Can you work these out from the model? Positions are in its coordinate system, mm. Face numbers are marked on the shaded views. Give positions to 0.01 mm unless a question says otherwise; leave off trailing zeros. Answer as a JSON object with one key per item and string values.
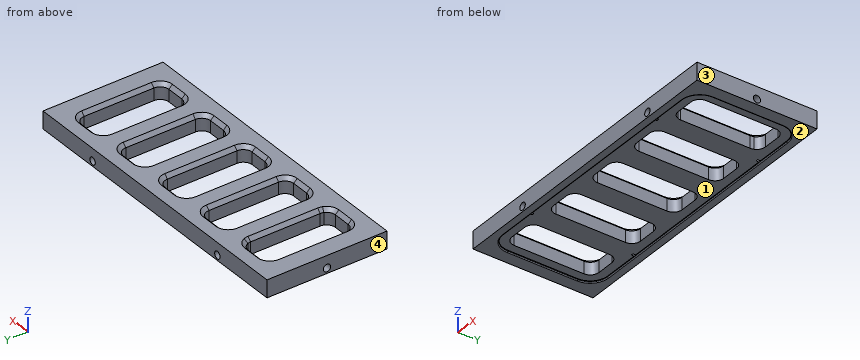
```python
from build123d import *

# Parameters (mm, degrees)
SKETCH_1_W           = 10
SKETCH_1_H           = 68.9
EXTRUDE_1_DEPTH      = 175
CUT_EXTRUDE_1_DEPTH  = 10
CHAMFER_1_SIZE       = 2
SKETCH_5_R           = 2.1
CUT_EXTRUDE_4_DEPTH  = 6
CUT_EXTRUDE_START    = -6
SKETCH_8_R           = 2.1
CUT_EXTRUDE_7_DEPTH  = 6
CUT_EXTRUDE_8_DEPTH  = 6
SKETCH_10_R          = 2.1
CUT_EXTRUDE_10_DEPTH = 6
CUT_EXTRUDE_11_DEPTH = 1
FILLET_1_R           = 0.5


with BuildPart() as part:
    # 草图1 → 凸台-拉伸1 (new body)
    with BuildSketch(Plane(origin=(0, 0, 0), x_dir=(0, 0, -1), z_dir=(1, 0, 0))):
        Rectangle(SKETCH_1_W, SKETCH_1_H)
    extrude(amount=EXTRUDE_1_DEPTH)

    # 草图2 → 切除-拉伸1 (cut)
    with BuildSketch(Plane.XY.offset(5)):
        Polygon((65, 8.858571429), (45, 16.732857143), (45, -16.732857143), (65, -8.858571429), align=None)
        with BuildLine():
            Line((45, 20), (45, 16.732857143))
            Line((45, 16.732857143), (65, 8.858571429))
            Line((65, 8.858571429), (65, 20))
            ThreePointArc((65, 20), (63.535533906, 23.535533906), (60, 25))
            Line((60, 25), (50, 25))
            ThreePointArc((50, 25), (46.464466094, 23.535533906), (45, 20))
        make_face()
        with BuildLine():
            Line((65, -8.858571429), (45, -16.732857143))
            Line((45, -16.732857143), (45, -20))
            ThreePointArc((45, -20), (46.464466094, -23.535533906), (50, -25))
            Line((50, -25), (60, -25))
            ThreePointArc((60, -25), (63.535533906, -23.535533906), (65, -20))
            Line((65, -20), (65, -8.858571429))
        make_face()
        with BuildLine():
            Line((32.170968927, -21.783829948), (24.002177068, -25))
            Line((24.002177068, -25), (27.5, -25))
            ThreePointArc((27.5, -25), (30.335564341, -24.118200441), (32.170968927, -21.783829948))
        make_face()
        with BuildLine():
            Line((32.170968927, 21.783829948), (24.002177068, 25))
            Line((24.002177068, 25), (17.5, 25))
            ThreePointArc((17.5, 25), (13.964466094, 23.535533906), (12.5, 20))
            Line((12.5, 20), (12.5, -20))
            ThreePointArc((12.5, -20), (13.964466094, -23.535533906), (17.5, -25))
            Line((17.5, -25), (24.002177068, -25))
            Line((24.002177068, -25), (32.170968927, -21.783829948))
            ThreePointArc((32.170968927, -21.783829948), (32.417054232, -20.906960684), (32.5, -20))
            Line((32.5, -20), (32.5, 20))
            ThreePointArc((32.5, 20), (32.417054232, 20.906960684), (32.170968927, 21.783829948))
        make_face()
        with BuildLine():
            Line((27.5, 25), (24.002177068, 25))
            Line((24.002177068, 25), (32.170968927, 21.783829948))
            ThreePointArc((32.170968927, 21.783829948), (30.335564341, 24.118200441), (27.5, 25))
        make_face()
        with BuildLine():
            Line((87.5, 0), (97.5, 3.937142857))
            Line((97.5, 3.937142857), (97.5, 20))
            ThreePointArc((97.5, 20), (96.035533906, 23.535533906), (92.5, 25))
            Line((92.5, 25), (82.5, 25))
            ThreePointArc((82.5, 25), (78.964466094, 23.535533906), (77.5, 20))
            Line((77.5, 20), (77.5, 3.937142857))
            Line((77.5, 3.937142857), (87.5, 0))
        make_face()
        Polygon((77.5, -3.937142857), (87.5, 0), (77.5, 3.937142857), align=None)
        with BuildLine():
            Line((97.5, -3.937142857), (87.5, 0))
            Line((87.5, 0), (77.5, -3.937142857))
            Line((77.5, -3.937142857), (77.5, -20))
            ThreePointArc((77.5, -20), (78.964466094, -23.535533906), (82.5, -25))
            Line((82.5, -25), (92.5, -25))
            ThreePointArc((92.5, -25), (96.035533906, -23.535533906), (97.5, -20))
            Line((97.5, -20), (97.5, -3.937142857))
        make_face()
        Polygon((97.5, -3.937142857), (97.5, 3.937142857), (87.5, 0), align=None)
        Polygon((130, -16.732857143), (130, 16.732857143), (110, 8.858571429), (110, -8.858571429), align=None)
        with BuildLine():
            Line((130, -20), (130, -16.732857143))
            Line((130, -16.732857143), (110, -8.858571429))
            Line((110, -8.858571429), (110, -20))
            ThreePointArc((110, -20), (111.464466094, -23.535533906), (115, -25))
            Line((115, -25), (125, -25))
            ThreePointArc((125, -25), (128.535533906, -23.535533906), (130, -20))
        make_face()
        with BuildLine():
            Line((110, 8.858571429), (130, 16.732857143))
            Line((130, 16.732857143), (130, 20))
            ThreePointArc((130, 20), (128.535533906, 23.535533906), (125, 25))
            Line((125, 25), (115, 25))
            ThreePointArc((115, 25), (111.464466094, 23.535533906), (110, 20))
            Line((110, 20), (110, 8.858571429))
        make_face()
        with BuildLine():
            Line((157.5, 25), (150.997822932, 25))
            Line((150.997822932, 25), (142.829031073, 21.783829948))
            ThreePointArc((142.829031073, 21.783829948), (142.582945768, 20.906960684), (142.5, 20))
            Line((142.5, 20), (142.5, -20))
            ThreePointArc((142.5, -20), (142.582945768, -20.906960684), (142.829031073, -21.783829948))
            Line((142.829031073, -21.783829948), (150.997822932, -25))
            Line((150.997822932, -25), (157.5, -25))
            ThreePointArc((157.5, -25), (161.035533906, -23.535533906), (162.5, -20))
            Line((162.5, -20), (162.5, 20))
            ThreePointArc((162.5, 20), (161.035533906, 23.535533906), (157.5, 25))
        make_face()
        with BuildLine():
            Line((142.829031073, 21.783829948), (150.997822932, 25))
            Line((150.997822932, 25), (147.5, 25))
            ThreePointArc((147.5, 25), (144.664435659, 24.118200441), (142.829031073, 21.783829948))
        make_face()
        with BuildLine():
            Line((147.5, -25), (150.997822932, -25))
            Line((150.997822932, -25), (142.829031073, -21.783829948))
            ThreePointArc((142.829031073, -21.783829948), (144.664435659, -24.118200441), (147.5, -25))
        make_face()
    extrude(amount=-CUT_EXTRUDE_1_DEPTH, mode=Mode.SUBTRACT)

    # 倒角1
    chamfer_1_edges = [part.edges().sort_by_distance(p)[0] for p in [
        (46.464466094, 23.535533906, 5),
        (55, 25, 5),
        (63.535533906, 23.535533906, 5),
        (55, -25, 5),
        (143.964466094, -23.535533906, 5),
        (142.5, 0, 5),
        (143.964466094, 23.535533906, 5),
        (152.5, 25, 5),
        (161.035533906, 23.535533906, 5),
        (162.5, 0, 5),
        (161.035533906, -23.535533906, 5),
        (152.5, -25, 5),
        (130, 0, 5),
        (128.535533906, -23.535533906, 5),
        (111.464466094, -23.535533906, 5),
        (110, 0, 5),
        (111.464466094, 23.535533906, 5),
        (120, 25, 5),
        (128.535533906, 23.535533906, 5),
        (120, -25, 5),
        (77.5, 0, 5),
        (78.964466094, 23.535533906, 5),
        (87.5, 25, 5),
        (96.035533906, 23.535533906, 5),
        (97.5, 0, 5),
        (96.035533906, -23.535533906, 5),
        (78.964466094, -23.535533906, 5),
        (87.5, -25, 5),
        (31.035533906, -23.535533906, 5),
        (13.964466094, -23.535533906, 5),
        (12.5, 0, 5),
        (13.964466094, 23.535533906, 5),
        (22.5, 25, 5),
        (31.035533906, 23.535533906, 5),
        (32.5, 0, 5),
        (22.5, -25, 5),
        (65, 0, 5),
        (63.535533906, -23.535533906, 5),
        (46.464466094, -23.535533906, 5),
        (45, 0, 5),
    ]]
    chamfer(chamfer_1_edges, length=CHAMFER_1_SIZE)

    # 草图5 → 切除-拉伸4 (cut)
    with BuildSketch(Plane(origin=(0, 34.45, 0), x_dir=(1, 0, 0), z_dir=(0, 1, 0))):
        with Locations(Location((38.75, 2, 0), (0, 0, 270))):
            Circle(SKETCH_5_R)
        with Locations(Location((136.25, 2, 0), (0, 0, 270))):
            Circle(SKETCH_5_R)
    extrude(amount=-CUT_EXTRUDE_4_DEPTH, mode=Mode.SUBTRACT)

    # 草图8 → 切除-拉伸7 (cut)
    with BuildSketch(Plane.XZ.offset(34.45).offset(CUT_EXTRUDE_START)):
        with Locations(Location((136.25, -2, 0), (0, 0, 90))):
            Circle(SKETCH_8_R)
        with Locations(Location((38.75, -2, 0), (0, 0, 90))):
            Circle(SKETCH_8_R)
    extrude(amount=CUT_EXTRUDE_7_DEPTH, mode=Mode.SUBTRACT)

    # 草图9 → 切除-拉伸8 (cut)
    with BuildSketch(Plane(origin=(175, 0, 0), x_dir=(0, 0, -1), z_dir=(1, 0, 0))):
        with BuildLine():
            ThreePointArc((4.1, 0), (2, 2.1), (-0.1, 0))
            Line((-0.1, 0), (4.1, 0))
        make_face()
        with BuildLine():
            Line((4.1, 0), (-0.1, 0))
            ThreePointArc((-0.1, 0), (2, -2.1), (4.1, 0))
        make_face()
    extrude(amount=-CUT_EXTRUDE_8_DEPTH, mode=Mode.SUBTRACT)

    # 草图10 → 切除-拉伸10 (cut)
    with BuildSketch(Plane.ZY.offset(CUT_EXTRUDE_START)):
        with Locations(Location((-2, 0, 0), (0, 0, 180))):
            Circle(SKETCH_10_R)
    extrude(amount=CUT_EXTRUDE_10_DEPTH, mode=Mode.SUBTRACT)

    # 草图11 → 切除-拉伸11 (cut)
    with BuildSketch(Plane(origin=(0, 0, -5), x_dir=(-1, 0, 0), z_dir=(0, 0, -1))):
        with BuildLine():
            Line((-157.5, 30), (-17.5, 30))
            ThreePointArc((-17.5, 30), (-10.428932188, 27.071067812), (-7.5, 20))
            Line((-7.5, 20), (-7.5, -20))
            ThreePointArc((-7.5, -20), (-10.428932188, -27.071067812), (-17.5, -30))
            Line((-17.5, -30), (-157.5, -30))
            ThreePointArc((-157.5, -30), (-164.571067812, -27.071067812), (-167.5, -20))
            Line((-167.5, -20), (-167.5, 20))
            ThreePointArc((-167.5, 20), (-164.571067812, 27.071067812), (-157.5, 30))
        make_face()
    extrude(amount=-CUT_EXTRUDE_11_DEPTH, mode=Mode.SUBTRACT)

    # 圆角1
    fillet_1_edges = [part.edges().sort_by_distance(p)[0] for p in [
        (10.428932188, -27.071067812, -5),
        (7.5, 0, -5),
        (10.428932188, 27.071067812, -5),
        (87.5, 30, -5),
        (164.571067812, 27.071067812, -5),
        (167.5, 0, -5),
        (164.571067812, -27.071067812, -5),
        (87.5, -30, -5),
    ]]
    fillet(fillet_1_edges, radius=FILLET_1_R)


solid = part.part
```
1) Imagine slicing it at A-A on y = 7. Give the number of separate pieces and of enclosed holes in the cut face, and give its area (3 significant figures).
Check sheet entries:
{"separate pieces": "6", "enclosed holes": "0", "area": "670 mm2"}
2) I need wall thicknesses on L1, parallel to X at y = -5, z = -2; L2, parallel to X at y = 16.5, z = -4.25; L3, parallel to Y at x = 60.5, z = -1.25. Which ranges of each line are inside material? Lowest first, please.
Check sheet entries:
{"L1": "0 to 12.5, 32.5 to 45, 65 to 77.5, 97.5 to 110, 130 to 142.5, 162.5 to 175", "L2": "0 to 7.5, 167.5 to 175", "L3": "-34.45 to -24.97, 24.97 to 34.45"}
3) I'm going to push flat-ended pins straight in: P1, Ø2, axis at x = 135.5, z = -1.5, coming from the +Y side; P2, Ø1.2, axis at x = 38.5, z = -1.5, coming from the -Y side; P3, Ø1, axis at x = 132, y = 10.5, coming from the -Z side. Where does each tip first touch, or does it pass through?
Check sheet entries:
{"P1": "y = 28.45", "P2": "y = -28.45", "P3": "z = -4"}
4) If we mould it in two halves opening along X, with no side actions, what happens to the marked faces 1, 2, 3 and 4? For each: released by +X, released by -X, zero draft, split by the parting line, or undercut.
Check sheet entries:
{"face 1": "undercut", "face 2": "zero draft", "face 3": "released by +X", "face 4": "released by -X"}
